Check sheet for the drawn part. Datum: minimum x, y, z corner. Units: mm. Round coordinates to 2 decimals unless told otherwise and drop trailing zeros. Write each loop counter-clockwise with the first axis right and the second up, starting at its lowest first coordinate (ties: lowest second). Pieces come first, ordered by that corner, then holes. Notation, with made-up numbers: M 69,50 L 119,50 A24 cw 119,67 Z; hole C -23,62 d5. An arc over 180 degrees is marked long. Put each result on its own line as item: value.
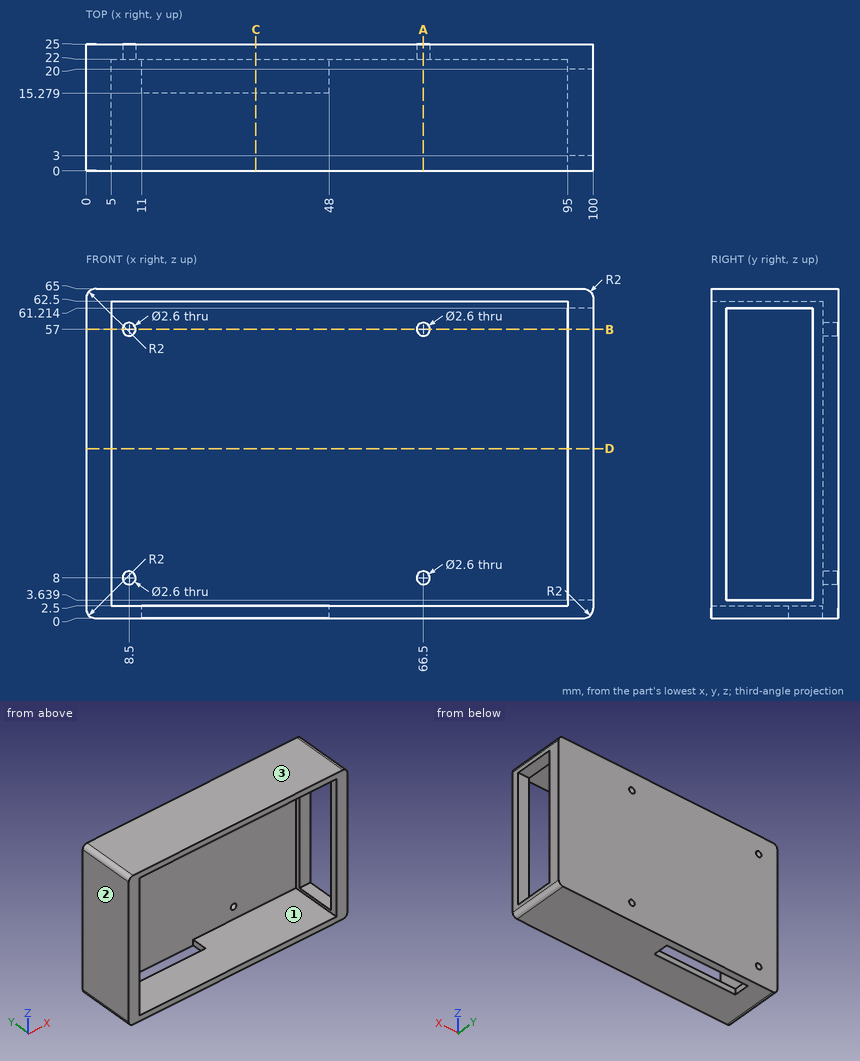
1. Cross-section at A-A (x = 66.5). Enter the section's corners in (y, z).
Computed values:
outline: M 0,0 L 25,0 L 25,6.7 L 22,6.7 L 22,2.5 L 0,2.5 Z; M 0,62.5 L 22,62.5 L 22,58.3 L 25,58.3 L 25,65 L 0,65 Z; M 22,9.3 L 25,9.3 L 25,55.7 L 22,55.7 Z
2. Cross-section at C-C (x = 33.5). Enter the section's corners in (y, z).
Computed values:
outline: M 0,0 L 15.28,0 L 15.28,2.5 L 0,2.5 Z; M 0,62.5 L 22,62.5 L 22,0 L 25,0 L 25,65 L 0,65 Z
3. Scan lines: probe 1 along Z at (x, y) = (66.5, 23.1); probe 2 along X at (y, z) = (23.95, 57); probe 3 along Z at (x, y) = (9.5, 12.75). Record each from-to range of solid material in increasing order.
Computed values:
probe 1: z = 0 to 6.7, 9.3 to 55.7, 58.3 to 65
probe 2: x = 0 to 7.2, 9.8 to 65.2, 67.8 to 100
probe 3: z = 0 to 2.5, 62.5 to 65
4. Cross-section at B-B (z = 57). Enter the section's corners in (x, y).
Computed values:
outline: M 0,0 L 5,0 L 5,22 L 7.2,22 L 7.2,25 L 0,25 Z; M 9.8,22 L 65.2,22 L 65.2,25 L 9.8,25 Z; M 67.8,22 L 95,22 L 95,20 L 100,20 L 100,25 L 67.8,25 Z; M 95,0 L 100,0 L 100,3 L 95,3 Z
5. Cross-section at D-D (z = 33.5). Enter the section's corners in (x, y), then the cut area to 3 significant figures.
Computed values:
outline: M 0,0 L 5,0 L 5,22 L 95,22 L 95,20 L 100,20 L 100,25 L 0,25 Z; M 95,0 L 100,0 L 100,3 L 95,3 Z
area: 435 mm2
6. Depth check by flat-ended pin: pin 1 Ø1.2 at (y, z) = (19.5, 1) entering from -X; pin 2 Ø19 at (x, z) = (68, 42.5) entering from -Y; pin 3 Ø4 at (y, z) = (9.5, 10) entering from +X. Enter the tip coordinate at first touch or a pass-through.
Computed values:
pin 1: stops at x = 0.04
pin 2: stops at y = 22
pin 3: stops at x = 5
7. Release check for a two-part mould opening along X. For the marked faces 1, 2 and 3 record: +X half, -X half, draft (parallel to the pull), parting line (faces both ways), or undercut.
Computed values:
face 1: undercut
face 2: -X half
face 3: draft
